The listing builds one solid part. Answer for the finished solid, in the listing's coordinates (mm). A direction names the side the tool comes from. Coordinates: 2 decimals unless noted, no trailing zeros. Write each loop counter-clockwise with the first axis right and the second up, starting at its lowest first coordinate (ties: lowest second). Pieces come first, ordered by that corner, then holes.
from build123d import *

# Parameters (mm, degrees)
SKETCH_1_W          = 40
SKETCH_1_H          = 55
SKETCH_1_R          = 1.65
EXTRUDE_1_DEPTH     = 5
EXTRUDE_2_DEPTH     = 3
SKETCH_3_R          = 1.65
CUT_EXTRUDE_1_DEPTH = 8.5
CUT_EXTRUDE_2_DEPTH = 2.5
FILLET_1_R          = 3


with BuildPart() as part:
    # 草图1 → 凸台-拉伸1 (new body)
    with BuildSketch(Plane(origin=(0, 0, 0), x_dir=(1, 0, 0), z_dir=(0, 1, 0))):
        Rectangle(SKETCH_1_W, SKETCH_1_H)
        with Locations((-16, 16)):
            Circle(SKETCH_1_R, mode=Mode.SUBTRACT)
        with Locations((16, 16)):
            Circle(SKETCH_1_R, mode=Mode.SUBTRACT)
        with Locations((16, -16)):
            Circle(SKETCH_1_R, mode=Mode.SUBTRACT)
        with Locations((-16, -16)):
            Circle(SKETCH_1_R, mode=Mode.SUBTRACT)
    extrude(amount=EXTRUDE_1_DEPTH)

    # 草图2 → 凸台-拉伸2 (add, symmetric)
    with BuildSketch(Plane(origin=(0, 0, 0), x_dir=(0, 0, -1), z_dir=(1, 0, 0))):
        Polygon((-18.5, 0), (-8.5, 0), (-11, -2.5), (-16, -2.5), align=None)
        Polygon((11, -2.5), (16, -2.5), (18.5, 0), (8.5, 0), align=None)
    extrude(amount=EXTRUDE_2_DEPTH, both=True)

    # 草图3 → 切除-拉伸1 (cut, through all)
    with BuildSketch(Plane(origin=(0, 5, 0), x_dir=(1, 0, 0), z_dir=(0, 1, 0))):
        with Locations((0, -24)):
            Circle(SKETCH_3_R)
        with Locations((0, 24)):
            Circle(SKETCH_3_R)
    extrude(amount=-CUT_EXTRUDE_1_DEPTH, mode=Mode.SUBTRACT)

    # 草图4 → 切除-拉伸2 (cut)
    with BuildSketch(Plane.XZ):
        Polygon((-14.383419246, 18.8), (-17.616580754, 18.8), (-19.233161507, 16), (-17.616580754, 13.2), (-14.383419246, 13.2), (-12.766838493, 16), align=None)
        Polygon((17.616580754, 18.8), (14.383419246, 18.8), (12.766838493, 16), (14.383419246, 13.2), (17.616580754, 13.2), (19.233161507, 16), align=None)
        Polygon((14.383419246, -13.2), (12.766838493, -16), (14.383419246, -18.8), (17.616580754, -18.8), (19.233161507, -16), (17.616580754, -13.2), align=None)
        Polygon((-17.616580754, -13.2), (-19.233161507, -16), (-17.616580754, -18.8), (-14.383419246, -18.8), (-12.766838493, -16), (-14.383419246, -13.2), align=None)
    extrude(amount=-CUT_EXTRUDE_2_DEPTH, mode=Mode.SUBTRACT)

    # 圆角1
    fillet_1_edges = [part.edges().sort_by_distance(p)[0] for p in [
        (20, 2.5, 27.5),
        (-20, 2.5, 27.5),
        (-20, 2.5, -27.5),
        (20, 2.5, -27.5),
    ]]
    fillet(fillet_1_edges, radius=FILLET_1_R)


solid = part.part
Q1. The part is cut by section A-A, the plane x = 0. Write down the section's boundary in (y, z).
Answers below:
outline: (-2.5, -16) - (0, -18.5) - (0, -22.35) - (5, -22.35) - (5, 22.35) - (0, 22.35) - (0, 18.5) - (-2.5, 16) - (-2.5, 11) - (0, 8.5) - (0, -8.5) - (-2.5, -11) - close; (0, -27.5) - (5, -27.5) - (5, -25.65) - (0, -25.65) - close; (0, 25.65) - (5, 25.65) - (5, 27.5) - (0, 27.5) - close
Q2. Which of the six approach directions +Z, -Z, +X, -X, +Y, -Y give full straight-line access (tool end or side, diameter ignored) to faces 1 (the face through (-18.414, 1.232, -14.58)), 2 (the face through (0, -1.3, 17.2)), 3 (the face through (0, -1.2, -9.7))?
Answers below:
face 1: -Y
face 2: +Z, +X, -X, -Y
face 3: +X, -X, -Y
Q3. Find the intervals of material crossed by probe 1 along Z at (x, y) = (16, 3.65); probe 2 along X at (y, z) = (4.05, -16); probe 3 along Y at (x, z) = (-15, 2), in increasing order.
Answers below:
probe 1: z = -27.5 to -17.65, -14.35 to 14.35, 17.65 to 27.5
probe 2: x = -20 to -17.65, -14.35 to 14.35, 17.65 to 20
probe 3: y = 0 to 5
Q4. The part is cut by section D-D, the plane y = -1. Write down the section's boundary in (x, z).
Answers below:
outline: (-3, -17.5) - (3, -17.5) - (3, -9.5) - (-3, -9.5) - close; (-3, 9.5) - (3, 9.5) - (3, 17.5) - (-3, 17.5) - close
Q5. Determine the mould class of faces 4 (the face through (0, 2, 27.5)), 5 (the face through (20, 2, 0)), 6 (the face through (-13.564, 1.232, 17.38)) for opening direction X: released by +X, released by -X, zero draft, split by the parting line, or undercut.
Answers below:
face 4: zero draft
face 5: released by +X
face 6: undercut
Q6. The part is cut by section C-C, the plane z = 15. Write down the section's boundary in (x, y).
Answers below:
outline: (-20, 0) - (-18.66, 0) - (-18.66, 2.5) - (-17.31, 2.5) - (-17.31, 5) - (-20, 5) - close; (-14.69, 2.5) - (-13.34, 2.5) - (-13.34, 0) - (-3, 0) - (-3, -2.5) - (3, -2.5) - (3, 0) - (13.34, 0) - (13.34, 2.5) - (14.69, 2.5) - (14.69, 5) - (-14.69, 5) - close; (17.31, 2.5) - (18.66, 2.5) - (18.66, 0) - (20, 0) - (20, 5) - (17.31, 5) - close
Q7. Given pin 1 (1.7 mm diameter, centred on x = -16.5, z = 15, fed in from -Y); pin 2 (1.5 mm diameter, centred on x = -11.5, z = 14, fed in from -Y); pin 3 (1.3 mm diameter, centred on y = -1.5, z = 13.5, fed in from -X), each flat-ended and moving along its own axis, determine where each tip first touches the part or whether it passes through.
Answers below:
pin 1: stops at y = 2.5
pin 2: stops at y = 0
pin 3: stops at x = -3
Q8. The part is cut by section B-B, the plane y = 3.25. Write down the section's boundary in (x, z).
Answers below:
outline: (-20, -24.5) arc R3 ccw to (-17, -27.5) - (17, -27.5) arc R3 ccw to (20, -24.5) - (20, 24.5) arc R3 ccw to (17, 27.5) - (-17, 27.5) arc R3 ccw to (-20, 24.5) - close; hole circle Ø3.3 at (-16, -16); hole circle Ø3.3 at (-16, 16); hole circle Ø3.3 at (0, -24); hole circle Ø3.3 at (0, 24); hole circle Ø3.3 at (16, -16); hole circle Ø3.3 at (16, 16)
